Part model, mm, in its own coordinate system. Coordinates: 2 decimals unless noted, no trailing zeros. Use a Markdown table: item, result. Add a question column.
1) Band-saw the part on A-A (y = 2.9). Give the number of separate pieces and of enclosed holes in the cut face, plus the area to 3 significant figures.
2) Drop flat-ended pins along their axis: P1, Ø1.8, axis at x = 159.34, z = -98.48, coming from the +Y side; P2, Ø3.5, axis at x = 5.84, z = -6.95, coming from the +Y side. Give the stop position or say it passes through.
3) Probe probe 1 along Z at (x, y) = (147, 0.6); probe 2 along X at (y, z) = (3.05, -234.5); probe 3 along X at (y, z) = (2.4, -222). List the from-to ranges inside material, lowest first. Write a range as [from, to].
from build123d import *

# Parameters (mm, degrees)
BOSS_EXTRUDE1_DEPTH = 5
SKETCH2_R           = 1.5
CUT_EXTRUDE1_DEPTH  = 10


with BuildPart() as part:
    # Sketch1 → Boss-Extrude1 (new body)
    with BuildSketch(Plane(origin=(0, 0, 0), x_dir=(1, 0, 0), z_dir=(0, 1, 0))):
        Polygon((0, 0), (151.72, 0), (165.843118786, 35.310315996), (165.843118786, 214.600315996), (151.72, 249.910631993), (0, 249.910631993), (-14.123118786, 214.600315996), (-14.123118786, 35.310315996), align=None)
    extrude(amount=BOSS_EXTRUDE1_DEPTH)

    # Sketch2 → Cut-Extrude1 (cut)
    with BuildSketch(Plane(origin=(0, 5, 0), x_dir=(1, 0, 0), z_dir=(0, 1, 0))):
        with Locations((159.339988978, 98.477853355)):
            Circle(SKETCH2_R)
        with Locations((145.883373815, 6.952127765)):
            Circle(SKETCH2_R)
        with Locations((5.840897433, 6.952127765)):
            Circle(SKETCH2_R)
        with Locations((-7.615717731, 98.477853355)):
            Circle(SKETCH2_R)
        with Locations((-7.615717731, 151.522146645)):
            Circle(SKETCH2_R)
        with Locations((5.840897433, 243.047872235)):
            Circle(SKETCH2_R)
        with Locations((145.883373815, 243.047872235)):
            Circle(SKETCH2_R)
        with Locations((159.339988978, 151.522146645)):
            Circle(SKETCH2_R)
    extrude(amount=-CUT_EXTRUDE1_DEPTH, mode=Mode.SUBTRACT)


solid = part.part
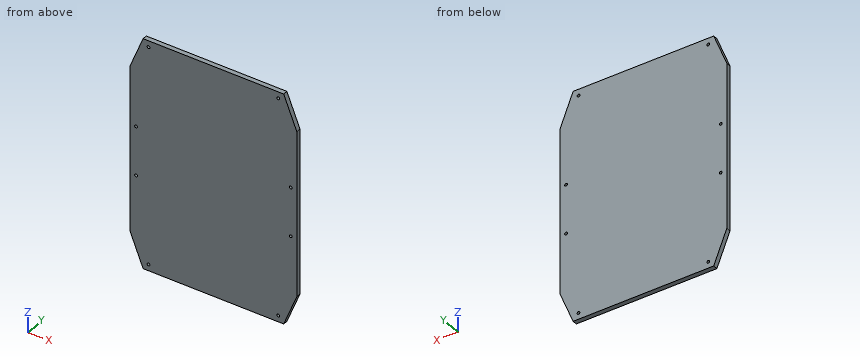
Answer block:
| question | item | result |
|---|---|---|
| 1 | separate pieces | 1 |
| 1 | enclosed holes | 8 |
| 1 | area | 43,900 mm2 |
| 2 | P1 | through |
| 2 | P2 | y = 5 |
| 3 | probe 1 | [-249.91, -244.05], [-242.05, -7.95], [-5.95, 0] |
| 3 | probe 2 | [-6.16, 157.88] |
| 3 | probe 3 | [-11.16, 162.88] |
